from build123d import *

# Parameters (mm, degrees)
SKETCH1_R               = 40
SKETCH1_R_2             = 25
BOSS_EXTRUDE1_DEPTH     = 61.9
CUT_EXTRUDE1_DEPTH      = 84.854695754
CUT_EXTRUDE1_DEPTH_BACK = 84.854695754
SKETCH2_W               = 16
SKETCH2_H               = 10


with BuildPart() as part:
    # Sketch1 → Boss-Extrude1 (new body)
    with BuildSketch(Plane(origin=(0, 0, 0), x_dir=(1, 0, 0), z_dir=(0, 1, 0))):
        with Locations(Location((0, 0, 0), (0, 0, 270))):
            Circle(SKETCH1_R)
        with Locations(Location((0, 0, 0), (0, 0, 270))):
            Circle(SKETCH1_R_2, mode=Mode.SUBTRACT)
    extrude(amount=BOSS_EXTRUDE1_DEPTH)

    # Sketch2 → Cut-Extrude1 (cut, two sides: drawn at the far end of the back side and taken through both)
    with BuildSketch(Plane(origin=(0, 61.9, 0), x_dir=(1, 0, 0), z_dir=(0, 1, 0)).offset(-CUT_EXTRUDE1_DEPTH_BACK)):
        with Locations((0, 25)):
            Rectangle(SKETCH2_W, SKETCH2_H)
    extrude(amount=CUT_EXTRUDE1_DEPTH + CUT_EXTRUDE1_DEPTH_BACK, mode=Mode.SUBTRACT)


solid = part.part
Source: CAD feature listing. Evaluate the final solid. Frame: model axes, mm. A direction names the side the tool comes from. Give positions to 0.01 mm unless a question says otherwise; leave off trailing zeros. Write each loop counter-clockwise with the first axis right and the second up, starting at its lowest first coordinate (ties: lowest second). Pieces come first, ordered by that corner, then holes. Notation, with made-up numbers: (-19, 12) - (22, 12) arc R26 cw to (22, 45) - close; hole circle Ø9 at (8.5, 14.5). An arc over 180 degrees is marked (long way). Write item = value, one per line. Start each with the question number.
Q1. Cut plane D-D, the plane x = -34.5. Return loops of the section in (y, z), then the cut area to 3 significant figures.
Q2. Material intervals for probe 1 along X at (y, z) = (14.5, 0); probe 2 along Z at (x, y) = (-2, 43.5); probe 3 along X at (y, z) = (35.5, -8), sorted ascending.
Q3. Cut plane A-A, the plane x = 0. Return loops of the section in (y, z).
Q4. Cut plane B-B, the plane z = 0. Return loops of the section in (x, y), then the cut area to 3 significant figures.
Q5. Cut plane C-C, the plane y = 26. Return loops of the section in (x, z), then the cut area to 3 significant figures.
Q6. Draft query along X for faces 3 (the flat face through (0, 31, -30)), 4 (the cylindrical face through (-39.05, 30.52, -8.67)), 5 (the flat face through (18.34, 61.9, 17.22)). Return one class per face: +X half, -X half, draft (parallel to the pull), parting line (faces both ways), or undercut.
Q7. Reachability of faces 1 (the flat face through (-8, 31, -27)), 2 (the flat face through (18.34, 0, 17.22)) from +Z, -Z, +X, -X, +Y, -Y: full face, straight path, thin tool, end or side. Return the list, or none.
Q8. Pin query (flat end, axial travel): pin 1 Ø1 at (y, z) = (7, 17) entering from +X; pin 2 Ø8 at (x, y) = (14.5, 18) entering from -Z; pin 3 Ø1.5 at (x, y) = (-22, 9) entering from +Z. Return the tip coordinate at first contact, or that it passes through.
Computed values:
q1.outline = (0, -20.24) - (61.9, -20.24) - (61.9, 20.24) - (0, 20.24) - close
q1.area = 2,510 mm²
q2.probe_1 = -40 to -25, 25 to 40
q2.probe_2 = -39.95 to -30, 24.92 to 39.95
q2.probe_3 = -39.19 to -23.69, 23.69 to 39.19
q3.outline = (0, -40) - (61.9, -40) - (61.9, -30) - (0, -30) - close; (0, 25) - (61.9, 25) - (61.9, 40) - (0, 40) - close
q4.outline = (-40, 0) - (-25, 0) - (-25, 61.9) - (-40, 61.9) - close; (25, 0) - (40, 0) - (40, 61.9) - (25, 61.9) - close
q4.area = 1,860 mm²
q5.outline = circle Ø80 at (0, 0); hole (-8, -30) - (8, -30) - (8, -23.69) arc R25 ccw (long way) to (-8, -23.69) - close
q5.area = 2,980 mm²
q6.face_3 = undercut
q6.face_4 = parting line
q6.face_5 = draft
q7.face_1 = +Y, -Y
q7.face_2 = +Z, -Z, +X, -X, -Y
q8.pin_1 = 36.44
q8.pin_2 = -38.6
q8.pin_3 = 33.89
